from build123d import *

# Parameters (mm, degrees)
ESQUISSE1_W             = 434
ESQUISSE1_H             = 220
ESQUISSE1_W_2           = 394
ESQUISSE1_H_2           = 180
BOSS_EXTRU_1_DEPTH      = 3
ESQUISSE2_W             = 10
ESQUISSE2_H             = 3
ESQUISSE2_W_2           = 2
ENL_V_MAT_EXTRU_1_DEPTH = 3
ESQUISSE3_R             = 1.75
ENL_V_MAT_EXTRU_2_DEPTH = 3


with BuildPart() as part:
    # Esquisse1 → Boss.-Extru.1 (new body)
    with BuildSketch(Plane.XY):
        Rectangle(ESQUISSE1_W, ESQUISSE1_H)
        Rectangle(ESQUISSE1_W_2, ESQUISSE1_H_2, mode=Mode.SUBTRACT)
    extrude(amount=BOSS_EXTRU_1_DEPTH)

    # Esquisse2 → Enlèv. mat.-Extru.1 (cut)
    with BuildSketch(Plane.XY.offset(3)):
        with Locations((-210, 108.5)):
            Rectangle(ESQUISSE2_W, ESQUISSE2_H)
        with Locations((-180, 108.5)):
            Rectangle(ESQUISSE2_W, ESQUISSE2_H)
        with Locations((-150, 108.5)):
            Rectangle(ESQUISSE2_W, ESQUISSE2_H)
        with Locations((-120, 108.5)):
            Rectangle(ESQUISSE2_W, ESQUISSE2_H)
        with Locations((-90, 108.5)):
            Rectangle(ESQUISSE2_W, ESQUISSE2_H)
        with Locations((-30, 108.5)):
            Rectangle(ESQUISSE2_W, ESQUISSE2_H)
        with Locations((30, 108.5)):
            Rectangle(ESQUISSE2_W, ESQUISSE2_H)
        with Locations((60, 108.5)):
            Rectangle(ESQUISSE2_W, ESQUISSE2_H)
        with Locations((90, 108.5)):
            Rectangle(ESQUISSE2_W, ESQUISSE2_H)
        with Locations((120, 108.5)):
            Rectangle(ESQUISSE2_W, ESQUISSE2_H)
        with Locations((150, 108.5)):
            Rectangle(ESQUISSE2_W, ESQUISSE2_H)
        with Locations((180, 108.5)):
            Rectangle(ESQUISSE2_W, ESQUISSE2_H)
        with Locations((210, 108.5)):
            Rectangle(ESQUISSE2_W, ESQUISSE2_H)
        with Locations((210, -108.5)):
            Rectangle(ESQUISSE2_W, ESQUISSE2_H)
        with Locations((180, -108.5)):
            Rectangle(ESQUISSE2_W, ESQUISSE2_H)
        with Locations((150, -108.5)):
            Rectangle(ESQUISSE2_W, ESQUISSE2_H)
        with Locations((90, -108.5)):
            Rectangle(ESQUISSE2_W, ESQUISSE2_H)
        with Locations((60, -108.5)):
            Rectangle(ESQUISSE2_W, ESQUISSE2_H)
        with Locations((-30, -108.5)):
            Rectangle(ESQUISSE2_W, ESQUISSE2_H)
        with Locations((-60, -108.5)):
            Rectangle(ESQUISSE2_W, ESQUISSE2_H)
        with Locations((-90, -108.5)):
            Rectangle(ESQUISSE2_W, ESQUISSE2_H)
        with Locations((-120, -108.5)):
            Rectangle(ESQUISSE2_W, ESQUISSE2_H)
        with Locations((-150, -108.5)):
            Rectangle(ESQUISSE2_W, ESQUISSE2_H)
        with Locations((-210, -108.5)):
            Rectangle(ESQUISSE2_W, ESQUISSE2_H)
        with Locations((-180, -108.5)):
            Rectangle(ESQUISSE2_W, ESQUISSE2_H)
        with Locations((-216, -108.5)):
            Rectangle(ESQUISSE2_W_2, ESQUISSE2_H)
        with Locations((-216, 108.5)):
            Rectangle(ESQUISSE2_W_2, ESQUISSE2_H)
        with Locations((-60, 108.5)):
            Rectangle(ESQUISSE2_W, ESQUISSE2_H)
        with Locations((0, 108.5)):
            Rectangle(ESQUISSE2_W, ESQUISSE2_H)
        with Locations((120, -108.5)):
            Rectangle(ESQUISSE2_W, ESQUISSE2_H)
        with Locations((30, -108.5)):
            Rectangle(ESQUISSE2_W, ESQUISSE2_H)
        with Locations((0, -108.5)):
            Rectangle(ESQUISSE2_W, ESQUISSE2_H)
        with Locations((216, 108.5)):
            Rectangle(ESQUISSE2_W_2, ESQUISSE2_H)
        with Locations((216, -108.5)):
            Rectangle(ESQUISSE2_W_2, ESQUISSE2_H)
    extrude(amount=-ENL_V_MAT_EXTRU_1_DEPTH, mode=Mode.SUBTRACT)

    # Esquisse3 → Enlèv. mat.-Extru.2 (cut)
    with BuildSketch(Plane.XY.offset(3)):
        with Locations((-207, 98.5)):
            Circle(ESQUISSE3_R)
        with Locations((-50.1, 98.5)):
            Circle(ESQUISSE3_R)
        with Locations((-207, -16.46)):
            Circle(ESQUISSE3_R)
    extrude(amount=-ENL_V_MAT_EXTRU_2_DEPTH, mode=Mode.SUBTRACT)


solid = part.part
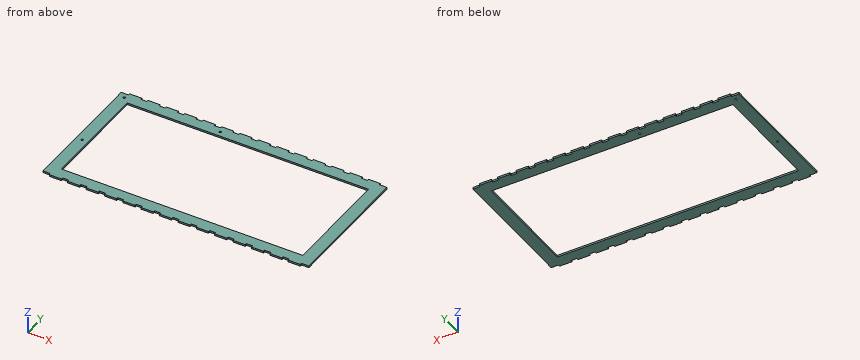
Verification items for the finished model (mm, model axes). Coordinates: 2 decimals unless noted, no trailing zeros. Write each loop counter-clockwise with the first axis right and the second up, starting at its lowest first coordinate (ties: lowest second). Pieces come first, ordered by that corner, then holes. Notation, with made-up numbers: (3, -38.5) -> (23, -38.5) arc R34 cw to (23, -5.5) -> close; hole circle Ø9 at (63.5, 12). An arc over 180 degrees is marked (long way). One line per item, written item: value. Start each with the question number.
Q1. Cross-section at B-B on x = -129.5. Enter the section's corners in (y, z), and give its area (3 significant figures).
Q2. Thickness scan on L1, parallel to Y at x = -50.1, z = 1.45; L2, parallel to Y at x = -207, z = 1.15; L3, parallel to X at y = 98.5, z = 1.1. Record the ranges inside material, lowest first. Write a range as from..to.
Q3. Cross-section at A-A on y = -66. Enter the section's corners in (x, z), and give its area (3 significant figures).
Q4. Cross-section at C-C on z = 0.95. State how many separate pieces and enclosed holes the cut face has, and give its area (3 significant figures).
Q5. Go/stop test with flat-tipped pins: P1, Ø1.5, axis at x = 90, z = 1.5, coming from the +Y side; P2, Ø1.5, axis at y = 108.5, z = 2, coming from the -X side; P3, Ø0.9, axis at y = -109, z = 2, coming from the +X side. Record where each tip stops, or that it passes through.
Checked values:
1. outline: (-110, 0) -> (-90, 0) -> (-90, 3) -> (-110, 3) -> close; (90, 0) -> (110, 0) -> (110, 3) -> (90, 3) -> close
1. area: 120 mm²
2. L1: y = -110..-90, 90..96.75, 100.25..110
2. L2: y = -107..-18.21, -14.71..96.75, 100.25..107
2. L3: x = -217..-208.75, -205.25..-51.85, -48.35..217
3. outline: (-217, 0) -> (-197, 0) -> (-197, 3) -> (-217, 3) -> close; (197, 0) -> (217, 0) -> (217, 3) -> (197, 3) -> close
3. area: 120 mm²
4. separate pieces: 1
4. enclosed holes: 4
4. area: 23,600 mm²
5. P1: stops at y = 107
5. P2: stops at x = -205
5. P3: stops at x = 205
